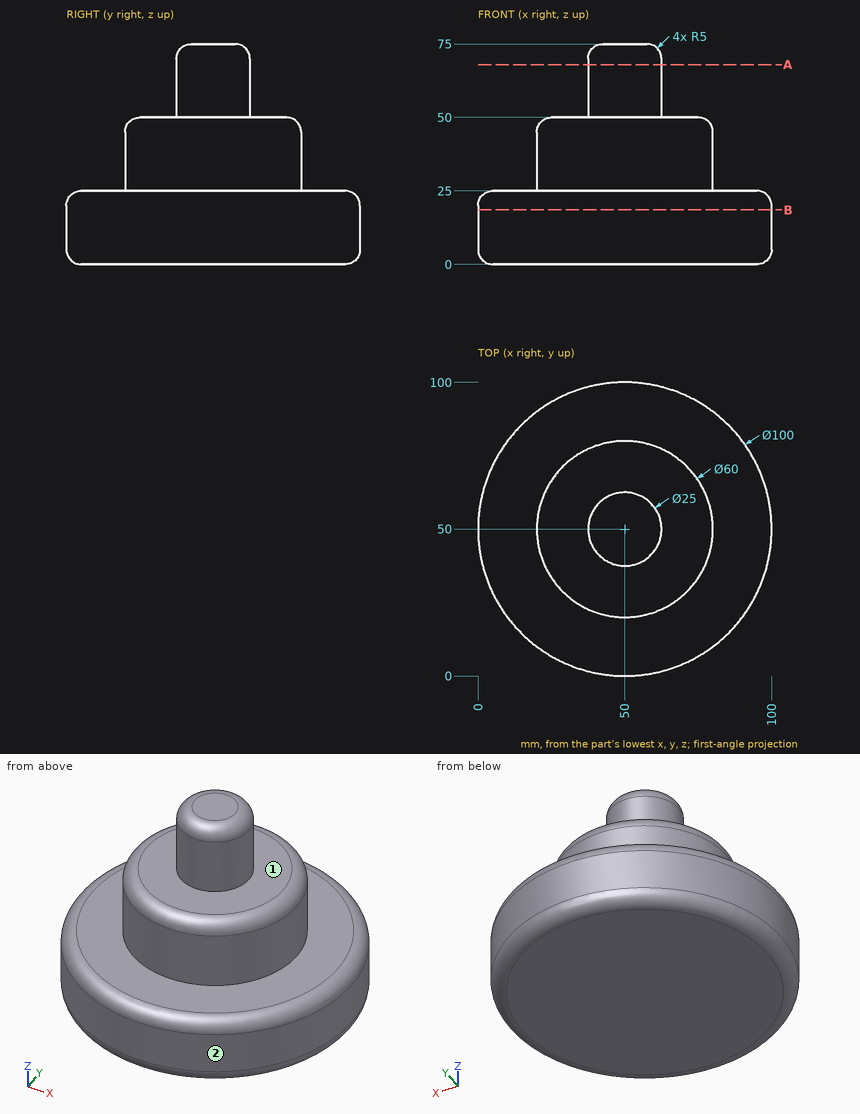
Study the drawing (mm; zero at the part's minimum x, y, z) and answer. A direction names the side the tool comes from. Give positions to 0.01 mm unless a question says otherwise; leave off trailing zeros. Write each loop counter-clockwise with the first axis right and the second up, starting at its lowest first coordinate (ties: lowest second). Pieces come first, ordered by that corner, then holes.
Item 1: Find the intervals of material crossed by line 1 along Z through (x, y) = (65.5, 85.5); line 2 along Z through (x, y) = (25.5, 52); line 3 along Y through (x, z) = (61, 35.5), in increasing order.
Item 2: Which of the six approach directions +Z, -Z, +X, -X, +Y, -Y give full straight-line access (tool end or side, diameter ignored) to the marked faces 1 and 2?
Item 3: Section A-A, the plane z = 68 is taken. Write down the section's boundary in (x, y).
Item 4: Section B-B, the plane z = 18.5 is taken. Write down the section's boundary in (x, y).
Item 5: Flat-ended cylindrical pins translate along their axes: P1, Ø1.5, axis at x = 21, z = 10, coming from the +Y side; P2, Ø1, axis at y = 41, z = 53.5, coming from the -X side; P3, Ø8, axis at x = 27.5, z = 24.5, coming from the -Y side. Find the tip coordinate at first contact, or state that the pin passes through.
Completed:
1. line 1: z = 0 to 25
1. line 2: z = 0 to 50
1. line 3: y = 22.09 to 77.91
2. face 1: +Z
2. face 2: +Z, -Z
3. outline: circle Ø25 at (50, 50)
4. outline: circle Ø100 at (50, 50)
5. P1: stops at y = 91.25
5. P2: stops at x = 40.83
5. P3: stops at y = 4.34
